Here's how the part is built. I have some questions about the finished solid (model axes, mm). Face numbers are marked on the shaded views. Coordinates: 2 decimals unless noted, no trailing zeros. Order: outer loops, then holes, each group sorted by start corner. A loop starts at its lowest first (then second) coordinate and runs counter-clockwise, first axis right, second up.
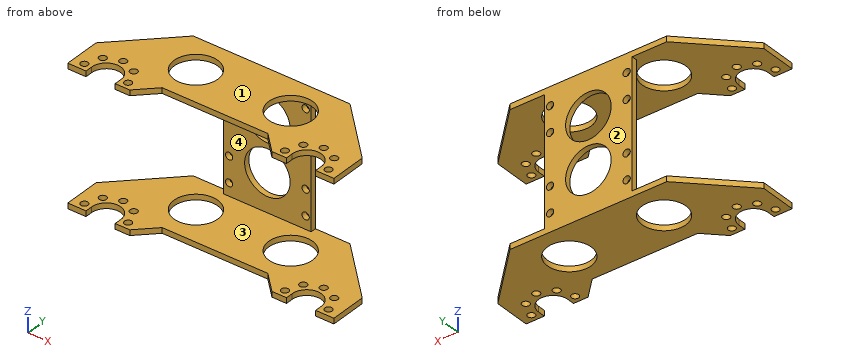
```python
from build123d import *

# Parameters (mm, degrees)
F0_R      = 1
F1_DEPTH  = 1.5
F3_DEPTH  = 1.5
F4_W      = 24
F4_H      = 1.5
F5_DEPTH  = 17.5
F8_R      = 6
F9_DEPTH  = 38.001
F10_R     = 1
F10_R_2   = 6.25
F11_DEPTH = 1.5


with BuildPart() as f1:
    # F0 (on Top) → F1 (new body)
    with BuildSketch(Plane.XY):
        with BuildLine():
            Line((-36.5, 25), (-36.5, 0))
            Line((-36.5, 0), (-31.5, 0))
            Line((-31.5, 0), (-31.5, 2))
            ThreePointArc((-31.5, 2), (-27.5, 6), (-23.5, 2))
            Line((-23.5, 2), (-23.5, 0))
            Line((-23.5, 0), (23.5, 0))
            Line((23.5, 0), (23.5, 2))
            ThreePointArc((23.5, 2), (27.5, 6), (31.5, 2))
            Line((31.5, 2), (31.5, 0))
            Line((31.5, 0), (36.5, 0))
            Line((36.5, 0), (36.5, 25))
            Line((36.5, 25), (-36.5, 25))
        make_face()
        with Locations((-33.5, 2)):
            Circle(F0_R, mode=Mode.SUBTRACT)
        with Locations((-21.5, 2)):
            Circle(F0_R, mode=Mode.SUBTRACT)
        with Locations((-31.742641, 6.242641)):
            Circle(F0_R, mode=Mode.SUBTRACT)
        with Locations((-23.257359, 6.242641)):
            Circle(F0_R, mode=Mode.SUBTRACT)
        with Locations((-27.5, 8)):
            Circle(F0_R, mode=Mode.SUBTRACT)
        with Locations((21.5, 2)):
            Circle(F0_R, mode=Mode.SUBTRACT)
        with Locations((33.5, 2)):
            Circle(F0_R, mode=Mode.SUBTRACT)
        with Locations((23.257359, 6.242641)):
            Circle(F0_R, mode=Mode.SUBTRACT)
        with Locations((31.742641, 6.242641)):
            Circle(F0_R, mode=Mode.SUBTRACT)
        with Locations((27.5, 8)):
            Circle(F0_R, mode=Mode.SUBTRACT)
    extrude(amount=F1_DEPTH)

    # F2 (on face) → F3 (cut, through all)
    with BuildSketch(Plane.XY.offset(1.5)):
        Polygon((-36.5, 25), (-36.5, 10), (-21.5, 25), align=None)
        Polygon((36.5, 25), (21.5, 25), (36.5, 10), align=None)
        Polygon((-14.5, 5), (-19.5, 0), (19.5, 0), (14.5, 5), (0, 5), align=None)
    extrude(amount=-F3_DEPTH, mode=Mode.SUBTRACT)

    # F4 (on face) → F5 (join)
    with BuildSketch(Plane(origin=(0, 0, 0), x_dir=(1, 0, 0), z_dir=(0, 0, -1))):
        with Locations((0, -24.25)):
            Rectangle(F4_W, F4_H)
    extrude(amount=F5_DEPTH)

    # F7: F1 across plane


with BuildPart() as f1_1:
    add(f1.part)
    add(f1.part.mirror(Plane.XY.offset(-17.5)))

    # F8 (on face) → F9 (cut, through all)
    with BuildSketch(Plane(origin=(0, 0, -36.5), x_dir=(1, 0, 0), z_dir=(0, 0, -1))):
        with Locations((-13, -15)):
            Circle(F8_R)
        with Locations((13, -15)):
            Circle(F8_R)
    extrude(amount=-F9_DEPTH, mode=Mode.SUBTRACT)

    # F10 (on face) → F11 (cut, through all)
    with BuildSketch(Plane(origin=(0, 25, 0), x_dir=(-1, 0, 0), z_dir=(0, 1, 0))):
        with Locations((10.5, -10.5)):
            Circle(F10_R)
        with Locations((10.5, -31.5)):
            Circle(F10_R)
        with Locations((-10.5, -10.5)):
            Circle(F10_R)
        with Locations((-10.5, -31.5)):
            Circle(F10_R)
        with Locations((0, -10.5)):
            Circle(F10_R_2)
        with Locations((-10.5, -24.5)):
            Circle(F10_R)
        with Locations((-10.5, -3.5)):
            Circle(F10_R)
        with Locations((10.5, -3.5)):
            Circle(F10_R)
        with Locations((10.5, -24.5)):
            Circle(F10_R)
        with Locations((0, -24.5)):
            Circle(F10_R_2)
    extrude(amount=-F11_DEPTH, mode=Mode.SUBTRACT)


solid = f1_1.part
```
Q1. If we section it at D-D on y = 21.75: Write out the boundary of the cut face in (x, z).
Q2. I need wall thicknesses on L1, parallel to Z at x = 10.5, y = 24.4; L2, parallel to Y at x = -27.5, z = 0.5; L3, parallel to Y at x = -13, z = -36.05. Which ranges of each line are inside material? Lowest first, please.
Q3. Will these pins go through, and if not, where does the flat tip stop? pin 1 (1.6 mm diameter, centred on x = -27.5, y = 8, fed in from -Z); pin 2 (6 mm diameter, centred on x = -10, z = -5.5, fed in from -Y); pin 3 (16 mm diameter, centred on x = 0, z = -24.5, fed in from +Y); pin 4 (1.2 mm diameter, centred on x = 2, z = -36, fed in from -Y).
Q4. If we section it at C-C on y = 8: Write out the boundary of the cut face in (x, z), then the cut area to 3 significant figures.
Q5. If we section it at A-A on z = -10.5: Write out the boundary of the cut face in (x, y).
Q6. If we section it at B-B on x = 0: Write out the boundary of the cut face in (y, z), then the cut area to 3 significant figures.
Q7. We'd pull the mould along Z, two halves only. Please class the marked faces 1, 2, 3 and 4: pulls with the +Z half, pulls with the -Z half, needs draft (parallel to the pull), parting line crosses it, or undercut.
Reply:
1. outline: (-24.75, -36.5) - (24.75, -36.5) - (24.75, -35) - (-24.75, -35) - close; (-24.75, 0) - (24.75, 0) - (24.75, 1.5) - (-24.75, 1.5) - close
2. L1: z = -36.5 to -32.5, -30.5 to -25.5, -23.5 to -11.5, -9.5 to -4.5, -2.5 to 1.5
2. L2: y = 6 to 7, 9 to 19
2. L3: y = 5 to 9, 21 to 25
3. pin 1: passes through
3. pin 2: stops at y = 23.5
3. pin 3: stops at y = 25
3. pin 4: stops at y = 5
4. outline: (-36.5, -36.5) - (-28.5, -36.5) - (-28.5, -35) - (-36.5, -35) - close; (-36.5, 0) - (-28.5, 0) - (-28.5, 1.5) - (-36.5, 1.5) - close; (-26.5, -36.5) - (26.5, -36.5) - (26.5, -35) - (-26.5, -35) - close; (-26.5, 0) - (26.5, 0) - (26.5, 1.5) - (-26.5, 1.5) - close; (28.5, -36.5) - (36.5, -36.5) - (36.5, -35) - (28.5, -35) - close; (28.5, 0) - (36.5, 0) - (36.5, 1.5) - (28.5, 1.5) - close
4. area: 207 mm2
5. outline: (-12, 23.5) - (-11.5, 23.5) - (-11.5, 25) - (-12, 25) - close; (-9.5, 23.5) - (-6.25, 23.5) - (-6.25, 25) - (-9.5, 25) - close; (6.25, 23.5) - (9.5, 23.5) - (9.5, 25) - (6.25, 25) - close; (11.5, 23.5) - (12, 23.5) - (12, 25) - (11.5, 25) - close
6. outline: (5, -36.5) - (25, -36.5) - (25, -30.75) - (23.5, -30.75) - (23.5, -35) - (5, -35) - close; (5, 0) - (23.5, 0) - (23.5, -4.25) - (25, -4.25) - (25, 1.5) - (5, 1.5) - close; (23.5, -18.25) - (25, -18.25) - (25, -16.75) - (23.5, -16.75) - close
6. area: 75.0 mm2
7. face 1: pulls with the +Z half
7. face 2: needs draft
7. face 3: undercut
7. face 4: undercut
